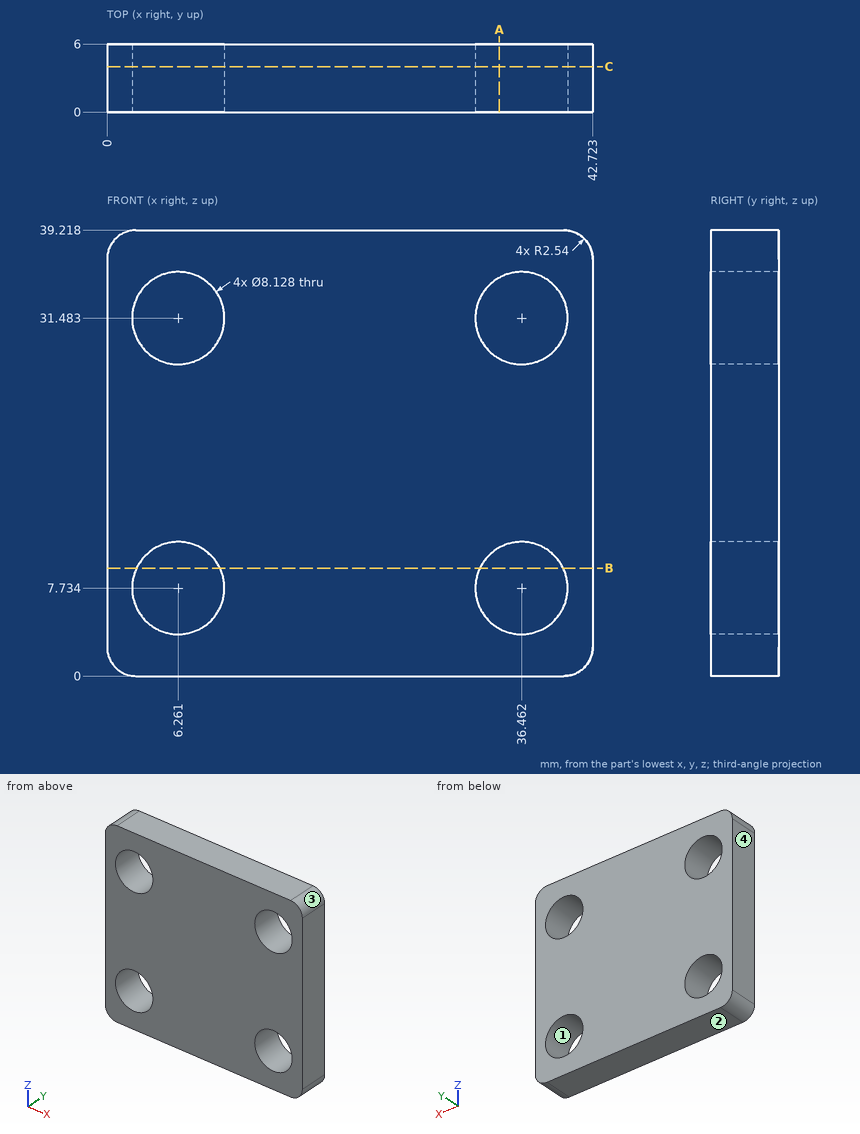
Check sheet for the drawn part. Datum: minimum x, y, z corner. Units: mm. Round coordinates to 2 decimals unless told otherwise and drop trailing zeros. Loops run counter-clockwise (first coordinate to the right, second up) from the corner with the lowest first, then second, coordinate; pieces in that order, holes last. Notation, with made-up numbers: (59, 42.25) - (79, 42.25) arc R6 ccw to (79, 46.25) - close; hole circle Ø5 at (66, 22.25). An arc over 180 degrees is marked (long way). Use one line per item in the form item = value.
1. Draft check along Z on the marked faces 1, 2, 3 and 4. Enter one of: pulls with the +Z half, pulls with the -Z half, needs draft (parallel to the pull), parting line crosses it, or undercut.
A:
face_1 = undercut
face_2 = pulls with the -Z half
face_3 = pulls with the +Z half
face_4 = needs draft
2. Section check A-A on x = 34.5. Record the cut outline in (y, z) (1 decimal), and give its area (3 significant figures).
A:
outline = (0, 0) - (6, 0) - (6, 4.2) - (0, 4.2) - close; (0, 11.3) - (6, 11.3) - (6, 27.9) - (0, 27.9) - close; (0, 35) - (6, 35) - (6, 39.2) - (0, 39.2) - close
area = 150 mm²
3. Section check C-C on y = 4. Record the cut outline in (x, z) (1 decimal).
A:
outline = (0, 2.5) arc R2.5 ccw to (2.5, 0) - (40.2, 0) arc R2.5 ccw to (42.7, 2.5) - (42.7, 36.7) arc R2.5 ccw to (40.2, 39.2) - (2.5, 39.2) arc R2.5 ccw to (0, 36.7) - close; hole circle Ø8.1 at (6.3, 7.7); hole circle Ø8.1 at (6.3, 31.5); hole circle Ø8.1 at (36.5, 7.7); hole circle Ø8.1 at (36.5, 31.5)
4. Gauge pin test, flat ends, axial feed: pin 1 Ø7.5 at (x, z) = (6.26, 7.73) entering from +Y; pin 2 Ø1 at (y, z) = (2.5, 26) entering from -X. Record the tip position at first contact, or that the pin passes through.
A:
pin_1 = through
pin_2 = 0
5. Scan lines: probe 1 along Z at (x, y) = (35.5, 1.75) (1 decimal); probe 2 along X at (y, z) = (5.5, 30.5) (1 decimal); probe 3 along X at (y, z) = (2.75, 33). Record each from-to range of solid material in increasing order.
A:
probe_1 = 0 to 3.8, 11.7 to 27.5, 35.4 to 39.2
probe_2 = 0 to 2.3, 10.2 to 32.5, 40.4 to 42.7
probe_3 = 0 to 2.49, 10.03 to 32.69, 40.23 to 42.72
6. Section check B-B on z = 9.5. Record the cut outline in (x, y).
A:
outline = (0, 0) - (2.6, 0) - (2.6, 6) - (0, 6) - close; (9.92, 0) - (32.8, 0) - (32.8, 6) - (9.92, 6) - close; (40.12, 0) - (42.72, 0) - (42.72, 6) - (40.12, 6) - close
